Answer from the drawing. Dimensions are ordinates in mm from the lowest x, y and z of the part. Coordinates: 2 decimals unless noted, no trailing zeros. Loops run counter-clockwise (first coordinate to the right, second up) from the corner with the lowest first, then second, coordinate; pieces in that order, holes last. Notation, with made-up numbers: (86, 69) -> (117, 69) arc R7 cw to (117, 76) -> close; hole circle Ø3 at (-4.5, 19). An arc over 180 degrees is marked (long way). Use a Markdown table: item, result.
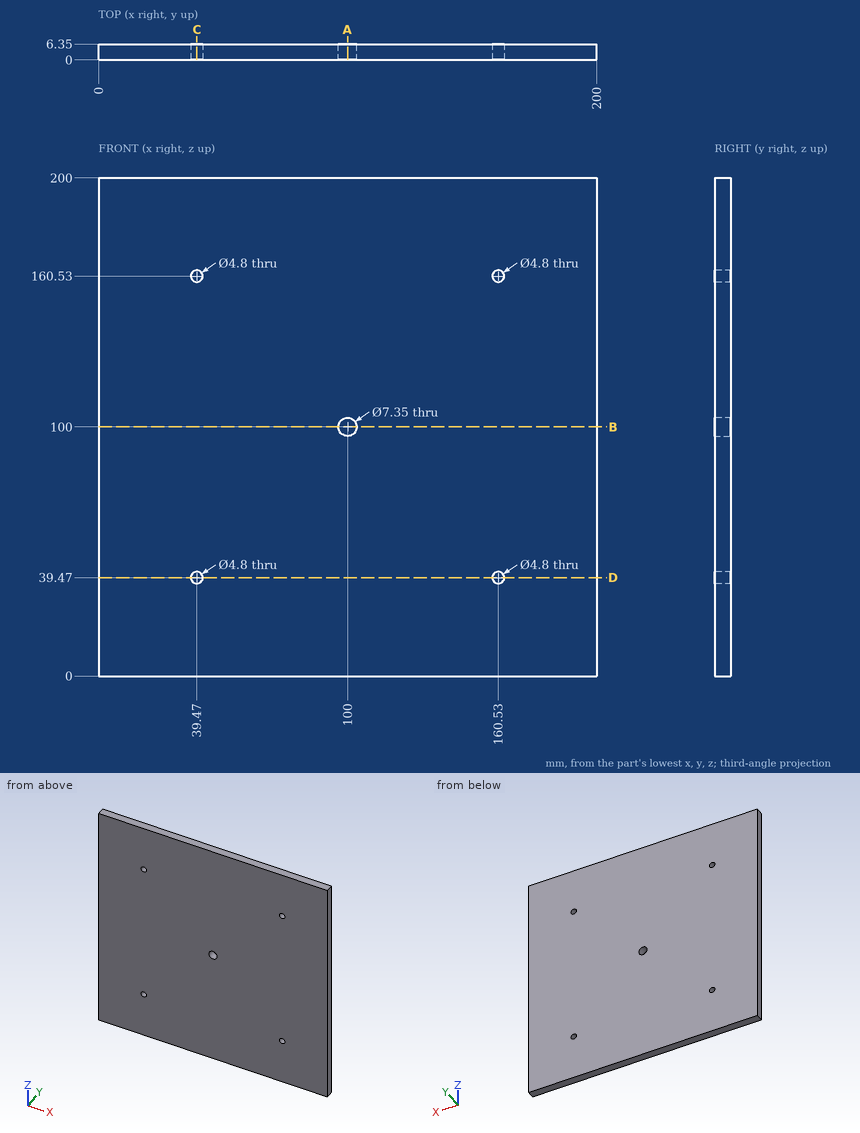
Q1. Section C-C on x = 39.47 is taken. Determine the outline of the cut face in (y, z), and give its area (3 significant figures).
Solved:
| item | result |
|---|---|
| outline | (0, 0) -> (6.35, 0) -> (6.35, 37.07) -> (0, 37.07) -> close; (0, 41.87) -> (6.35, 41.87) -> (6.35, 158.13) -> (0, 158.13) -> close; (0, 162.93) -> (6.35, 162.93) -> (6.35, 200) -> (0, 200) -> close |
| area | 1,210 mm² |
Q2. Given pin 1 Ø4.5 at (x, z) = (160.53, 39.47) entering from +Y, flat-ended and moving along its own axis, determine where the tip first touches the part or whether it passes through.
Solved:
| item | result |
|---|---|
| pin 1 | through |
Q3. Section D-D on z = 39.47 is taken. Determine the outline of the cut face in (x, y), and give its area (3 significant figures).
Solved:
| item | result |
|---|---|
| outline | (0, 0) -> (37.07, 0) -> (37.07, 6.35) -> (0, 6.35) -> close; (41.87, 0) -> (158.13, 0) -> (158.13, 6.35) -> (41.87, 6.35) -> close; (162.93, 0) -> (200, 0) -> (200, 6.35) -> (162.93, 6.35) -> close |
| area | 1,210 mm² |
Q4. Consider line 1 (X direction, y = 3, z = 39.47); line 2 (X direction, y = 3.5, z = 100) (3 decimals). Determine where each line is inside the solid, lowest interval first. Write a range as [from, to].
Solved:
| item | result |
|---|---|
| line 1 | [0, 37.07], [41.87, 158.13], [162.93, 200] |
| line 2 | [0, 96.325], [103.675, 200] |
Q5. Section A-A on x = 100 is taken. Determine the outline of the cut face in (y, z) (3 decimals), and give its area (3 significant figures).
Solved:
| item | result |
|---|---|
| outline | (0, 0) -> (6.35, 0) -> (6.35, 96.325) -> (0, 96.325) -> close; (0, 103.675) -> (6.35, 103.675) -> (6.35, 200) -> (0, 200) -> close |
| area | 1,220 mm² |
Q6. Section B-B on z = 100 is taken. Determine the outline of the cut face in (x, y) (3 decimals), and give its area (3 significant figures).
Solved:
| item | result |
|---|---|
| outline | (0, 0) -> (96.325, 0) -> (96.325, 6.35) -> (0, 6.35) -> close; (103.675, 0) -> (200, 0) -> (200, 6.35) -> (103.675, 6.35) -> close |
| area | 1,220 mm² |
